Here's how the part is built. I have some questions about the finished solid (model axes, mm). Round coordinates to 2 decimals unless told otherwise and drop trailing zeros. Order: outer loops, then holes, each group sorted by start corner. A loop starts at its lowest first (then second) coordinate and runs counter-clockwise, first axis right, second up. Notation, with made-up numbers: (-40, 63.5) -> (-35, 63.5) arc R13 ccw to (-35, 70.5) -> close; hole circle Ø10 at (39.25, 21.25). An arc over 180 degrees is marked (long way). Use a Markdown table: item, result. Add a question column.
Autodesk Inventor part; units mm, degrees
ref_plane "YZ Plane" through (0, 0, 0) normal (1, 0, 0) x (0, 1, 0)
ref_plane "XZ Plane" through (0, 0, 0) normal (0, 1, 0) x (-1, 0, 0)
ref_plane "XY Plane" through (0, 0, 0) normal (0, 0, 1) x (1, 0, 0)
sketch "Sketch1" plane through (0, 0, 0) normal (0, 1, 0) x (-1, 0, 0)
  line L0 (26.5, 66) -> (21.5, 66)
  line L1 (0, 63) -> (21.5, 63)
  line L2 (21.5, 63) -> (21.5, 66)
  line L3 (26.5, 66) -> (26.5, 63)
  line L4 (26.5, 63) -> (48, 63)
  line L5 (14, 0) -> (14, 3)
  line L6 (14, 3) -> (34, 3)
  line L7 (34, 3) -> (34, 0)
  line L8 (8, 0) -> (14, 0)
  line L9 (34, 0) -> (40, 0)
  line L10 (0, 63) -> (0, 38)
  line L11 (0, 28) -> (0, 3)
  line L12 (48, 3) -> (48, 28)
  line L13 (48, 38) -> (48, 63)
  line L14 (0, 38) -> (3, 38)
  line L15 (3, 38) -> (3, 28)
  line L16 (3, 28) -> (0, 28)
  line L17 (48, 38) -> (45, 38)
  line L18 (45, 38) -> (45, 28)
  line L19 (45, 28) -> (48, 28)
  line L20 (0, 3) -> (8, 3)
  line L21 (8, 3) -> (8, 0)
  line L22 (40, 3) -> (40, 0)
  line L23 (40, 3) -> (48, 3)
  point P0 (0, 0)
  dimension "d0" = 48
  dimension "d3" = 5
  dimension "d5" = 3
  dimension "d6" = 3
  dimension "d8" = 3
  dimension "d9" = 3
  dimension "d16" = 66
  dimension "d23" = 3
  dimension "d24" = 10
  dimension "d25" = 10
  dimension "d26" = 3
  dimension "d27" = 28
  dimension "d29" = 3
  dimension "d30" = 3
  dimension "d34" = 21.5
  dimension "d35" = 8
  dimension "d36" = 8
  dimension "d37" = 3
  dimension "d38" = 3
  dimension "d40" = 6
  dimension "d41" = 6
  dimension "d42" = 25
  dimension "d43" = 25
extrude "Extrusion1" add sketch "Sketch1" along normal blind 3
properties part number "Bottom"
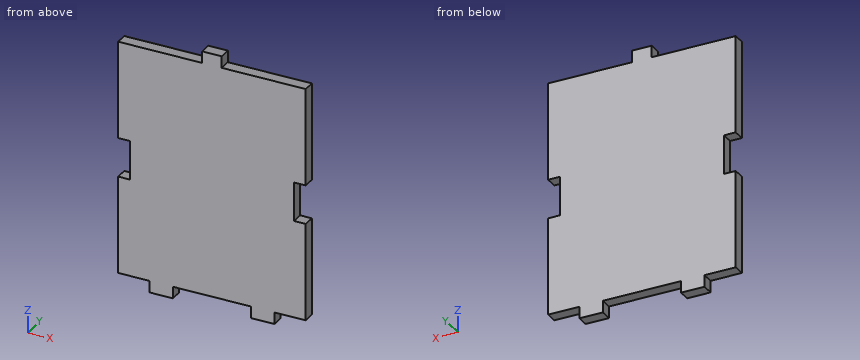
(1) I'm going to push flat-ended pins straight in: P1, Ø1.5, axis at x = -15.5, z = 39, coming from the -Y side; P2, Ø0.9, axis at y = 1.5, z = 2, coming from the -X side; P3, Ø1, axis at x = -41, y = 1, coming from the -Z side; P4, Ø1.5, axis at x = -13.5, y = 1, coming from the +Z side. Where does each tip first touch, or does it pass through?
(2) Please list where these lines run through material, in increasing order: probe 1 along X at (y, z) = (1.85, 29); probe 2 along Z at (x, y) = (-7, 2); probe 3 along Z at (x, y) = (-9.5, 0.95). Write a range as from..to.
(3) I want a section at B-B on x = -25. List the corners of the cut face in (y, z) for me.
(4) I want a section at A-A on y = 0.65. List the corners of the cut face in (x, z) for me.
(5) I want a section at C-C on z = 31.5. List the corners of the cut face in (x, y) for me.
Output:
| question | item | result |
|---|---|---|
| 1 | P1 | y = 0 |
| 1 | P2 | x = -40 |
| 1 | P3 | z = 3 |
| 1 | P4 | z = 63 |
| 2 | probe 1 | -45..-3 |
| 2 | probe 2 | 3..63 |
| 2 | probe 3 | 0..63 |
| 3 | outline | (0, 3) -> (3, 3) -> (3, 66) -> (0, 66) -> close |
| 4 | outline | (-48, 3) -> (-40, 3) -> (-40, 0) -> (-34, 0) -> (-34, 3) -> (-14, 3) -> (-14, 0) -> (-8, 0) -> (-8, 3) -> (0, 3) -> (0, 28) -> (-3, 28) -> (-3, 38) -> (0, 38) -> (0, 63) -> (-21.5, 63) -> (-21.5, 66) -> (-26.5, 66) -> (-26.5, 63) -> (-48, 63) -> (-48, 38) -> (-45, 38) -> (-45, 28) -> (-48, 28) -> close |
| 5 | outline | (-45, 0) -> (-3, 0) -> (-3, 3) -> (-45, 3) -> close |
